Part model, mm, in its own coordinate system. Face numbers are marked on the shaded views. A direction names the side the tool comes from. Round coordinates to 2 decimals unless told otherwise and drop trailing zeros. Loops run counter-clockwise (first coordinate to the right, second up) from the corner with the lowest first, then second, coordinate; pieces in that order, holes last.
1) Band-saw the part on D-D, the plane x = 42. Write the cut outline in (y, z), then the cut area to 3 significant figures.
2) Band-saw the part on C-C, the plane y = 57. Write the cut outline in (x, z), then the cut area to 3 significant figures.
3) Mould opens along Y. For the marked faces 4, 5, 6 and 7 say: +Y half, -Y half, draft (parallel to the pull), parting line (faces both ways), or undercut.
4) Drop flat-ended pins along their axis: P1, Ø5, axis at y = 7.5, z = 9, coming from the +X side; P2, Ø6.5, axis at x = 25, z = 10, coming from the -Y side; P3, Ø8, axis at y = 55.5, z = 13.5, coming from the +X side. Give the stop position or say it passes through.
5) Band-saw the part on A-A, the plane z = 1.5. Write the cut outline in (x, y).
6) Band-saw the part on B-B, the plane y = 109.5. Write the cut outline in (x, z), then the cut area to 3 significant figures.
7) Probe line 1 (Z direction, x = 8, y = 12); line 2 (X direction, y = 88, z = 14); line 3 (Y direction, x = 103, z = 12.5). List the from-to ranges inside material, lowest first.
8) 3-axis set-ups, long thin cutter, end or side, ignore diameter. For the marked faces 1, 2 and 3: which of +Z, -Z, +X, -X, +Y, -Y reach the whole face in a straight line?
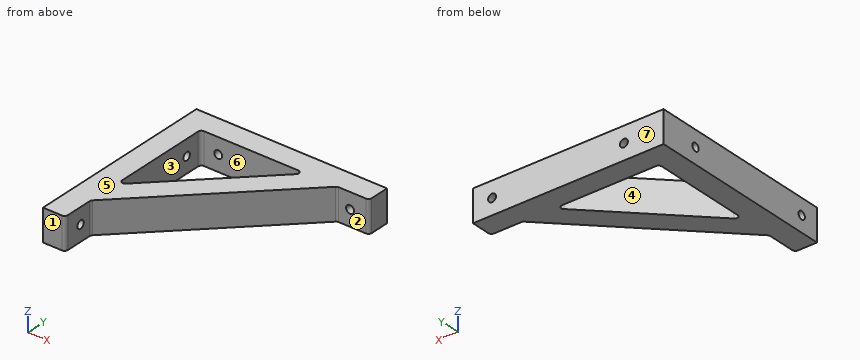
from build123d import *

# Parameters (mm, degrees)
F1_DEPTH = 20
F2_R     = 2.5
F3_DEPTH = 25
F4_R     = 2.5
F5_DEPTH = 25
F6_R     = 2


with BuildPart() as f1:
    # F0 (on Top) → F1 (new body)
    with BuildSketch(Plane.XY):
        Polygon((0, 120), (0, 0), (14, 0), (14, 20), (100, 106), (120, 106), (120, 120), align=None)
        Polygon((14, 39.79899), (14, 106), (80.20101, 106), align=None, mode=Mode.SUBTRACT)
    extrude(amount=F1_DEPTH)

    # F2 (on face) → F3 (cut)
    with BuildSketch(Plane(origin=(0, 0, 0), x_dir=(0, -1, 0), z_dir=(-1, 0, 0))):
        with Locations((-12, 10)):
            Circle(F2_R)
        with Locations((-95, 10)):
            Circle(F2_R)
    extrude(amount=-F3_DEPTH, mode=Mode.SUBTRACT)

    # F4 (on face) → F5 (cut)
    with BuildSketch(Plane(origin=(0, 120, 0), x_dir=(-1, 0, 0), z_dir=(0, 1, 0))):
        with Locations((-108, 10)):
            Circle(F4_R)
        with Locations((-25, 10)):
            Circle(F4_R)
    extrude(amount=-F5_DEPTH, mode=Mode.SUBTRACT)

    # F6
    f6_edges = [f1.edges().sort_by_distance(p)[0] for p in [
        (14, 39.79899, 10),
        (14, 106, 10),
        (80.20101, 106, 10),
        (14, 20, 10),
        (100, 106, 10),
        (120, 106, 10),
        (14, 0, 10),
    ]]
    fillet(f6_edges, radius=F6_R)


solid = f1.part
Reported:
1. outline: (48, 0) - (67.8, 0) - (67.8, 20) - (48, 20) - close; (106, 0) - (120, 0) - (120, 20) - (106, 20) - close
1. area: 676 mm2
2. outline: (0, 0) - (14, 0) - (14, 20) - (0, 20) - close; (31.2, 0) - (51, 0) - (51, 20) - (31.2, 20) - close
2. area: 676 mm2
3. face 4: undercut
3. face 5: draft
3. face 6: undercut
3. face 7: +Y half
4. P1: stops at x = 14
4. P2: stops at y = 27.75
4. P3: stops at x = 53.5
5. outline: (0, 0) - (12, 0) arc R2 ccw to (14, 2) - (14, 19.17) arc R2 cw to (14.59, 20.59) - (99.41, 105.41) arc R2 cw to (100.83, 106) - (118, 106) arc R2 ccw to (120, 108) - (120, 120) - (0, 120) - close; hole (14, 44.63) arc R2 ccw to (17.41, 43.21) - (76.79, 102.59) arc R2 ccw to (75.37, 106) - (16, 106) arc R2 ccw to (14, 104) - close
6. outline: (0, 0) - (120, 0) - (120, 20) - (0, 20) - close; hole circle Ø5 at (25, 10); hole circle Ø5 at (108, 10)
6. area: 2,360 mm2
7. line 1: z = 0 to 7.5, 12.5 to 20
7. line 2: x = 0 to 14, 62.2 to 82
7. line 3: y = 106 to 120
8. face 1: +Z, -Z, +X, -X, -Y
8. face 2: +Z, -Z, +X, -Y
8. face 3: +Z, -Z
